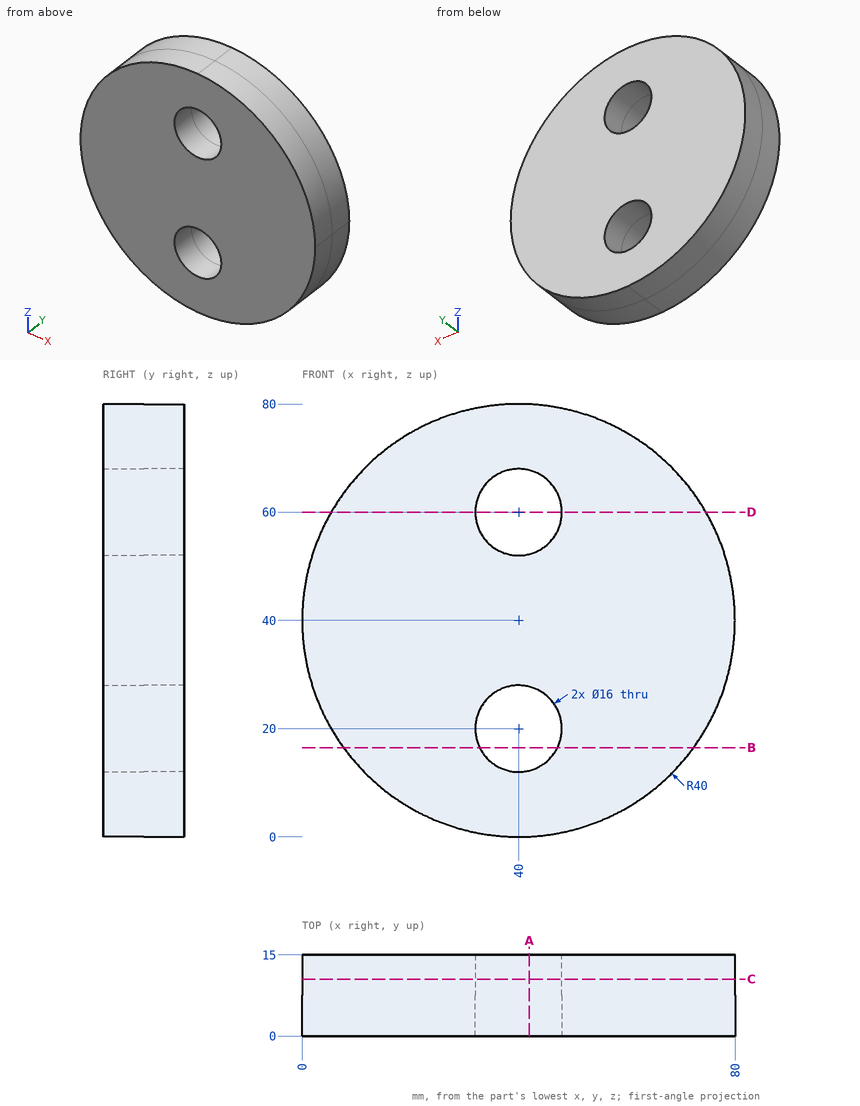
The figure shows three views and two pictorial views of one solid part (mm, origin at its lowest corner). Answer the questions. Give positions to 0.01 mm unless a question says otherwise; leave off trailing zeros. Order: outer loops, then holes, each group sorted by start corner. A loop starts at its lowest first (then second) coordinate and runs counter-clockwise, first axis right, second up. Notation, with made-up numbers: M 78.5,25.5 L 126.5,25.5 A28 cw 126.5,47.5 Z; hole C -3.5,74.25 d2. An arc over 180 degrees is marked long. Return JSON: item names as keys, results as strings.
1) Each of these flat-tipped pins is pushed along its axis until it touches: pin 1 (6 mm diameter, centred on x = 71, y = 11, fed in from -Z); pin 2 (14.5 mm diameter, centred on x = 40, z = 20, fed in from -Y); pin 3 (1 mm diameter, centred on y = 10, z = 34.5, fed in from +X); pin 4 (5 mm diameter, centred on x = 66, y = 4.5, fed in from -Z). Where does it stop, or does it pass through?
Resolved:
{"pin 1": "z = 11.43", "pin 2": "through", "pin 3": "x = 79.69", "pin 4": "z = 7.63"}
2) Section C-C, the plane y = 10.5 is taken. Write down the section's boundary in (x, z), plus the area to 3 significant figures.
Resolved:
{"outline": "C 40,40 d80; hole C 40,20 d16; hole C 40,60 d16", "area": "4,620 mm^2"}
3) Straight lines are drawn through the part: line 1 along Z through (x, y) = (40, 12.25); line 2 along Z through (x, y) = (33, 12); line 3 along X through (y, z) = (7.75, 23.5). For each, find the intervals that lie inside material, in ascending order. Write a range as [from, to].
Resolved:
{"line 1": "[0, 12], [28, 52], [68, 80]", "line 2": "[0.62, 16.13], [23.87, 56.13], [63.87, 79.38]", "line 3": "[3.56, 32.81], [47.19, 76.44]"}
4) Section A-A, the plane x = 42 is taken. Write down the section's boundary in (y, z), plus the area to 3 significant figures.
Resolved:
{"outline": "M 0,0.05 L 15,0.05 L 15,12.25 L 0,12.25 Z; M 0,27.75 L 15,27.75 L 15,52.25 L 0,52.25 Z; M 0,67.75 L 15,67.75 L 15,79.95 L 0,79.95 Z", "area": "734 mm^2"}
5) Section D-D, the plane z = 60 is taken. Write down the section's boundary in (x, y), plus the area to 3 significant figures.
Resolved:
{"outline": "M 5.36,0 L 32,0 L 32,15 L 5.36,15 Z; M 48,0 L 74.64,0 L 74.64,15 L 48,15 Z", "area": "799 mm^2"}
6) Section B-B, the plane z = 16.5 is taken. Write down the section's boundary in (x, y), plus the area to 3 significant figures.
Resolved:
{"outline": "M 7.63,0 L 32.81,0 L 32.81,15 L 7.63,15 Z; M 47.19,0 L 72.37,0 L 72.37,15 L 47.19,15 Z", "area": "755 mm^2"}
